Geometry: final body of the model. Coordinates: model frame, mm. Face numbers are marked on the shaded views. A direction names the side the tool comes from. Give positions to 0.01 mm unless a question says otherwise; leave off trailing zeros. Write each loop counter-clockwise with the first axis right and the second up, starting at its lowest first coordinate (ties: lowest second). Pieces come first, ordered by that corner, then holes. Notation, with made-up numbers: M -4.75,-31 L 5.25,-31 A21 ccw 5.25,8 Z; hole C 42,56 d11. An arc over 180 degrees is marked long. Use a Markdown table: item, result. Add a question column.
(1) Material intervals for L1, parallel to X at y = 13.25, z = -20; L2, parallel to X at y = 6.5, z = -23; L3, parallel to Y at x = -16, z = -36.5, sorted ascending.
(2) Cut plane A-A (z = -52). Output: boundary loops of the cut face in (x, y), plus the area to 3 significant figures.
(3) Reachability of the marked faces 1, 2, 3, 4 and 5 from +Z, -Z, +X, -X, +Y, -Y: full face, straight path, thin tool, end or side. Return the list, or none.
(4) Cut plane D-D (z = -36). Output: boundary loops of the cut face in (x, y), plus the area to 3 significant figures.
(5) Cut plane C-C (y = 93). Output: boundary loops of the cut face in (x, z), plus the area to 3 significant figures.
(6) Cut plane B-B (x = -72). Output: boundary loops of the cut face in (y, z), plus the area to 3 significant figures.
(7) Pin query (flat end, axial travel): pin 1 Ø5 at (y, z) = (49.5, -51.5) entering from +X; pin 2 Ø19 at (y, z) = (46, -19.5) entering from +X; pin 3 Ø5 at (y, z) = (37.5, -32.5) entering from -X. Return the tip coordinate at first contact, or that it passes through.
(8) Draft query along X for the marked faces 6, 7, 8 and 9. Return one class per face: released by +X, released by -X, zero draft, split by the parting line, or undercut.
```python
from build123d import *

# Parameters (mm, degrees)
SKETCH2_R           = 10
BOSS_EXTRUDE1_DEPTH = 20
SKETCH3_W           = 120
SKETCH3_H           = 8
CUT_EXTRUDE1_DEPTH  = 4
SKETCH7_R           = 10
BOSS_EXTRUDE2_DEPTH = 16
BOSS_EXTRUDE3_START = 8
SKETCH8_R           = 24
SKETCH8_R_2         = 10
BOSS_EXTRUDE3_DEPTH = 8
RIB4_REACH          = 153.895
SKETCH9_WALL_W      = 381.261249794
SKETCH9_WALL_H      = 12
FILLET2_R           = 1


with BuildPart() as part:
    # Sketch2 → Boss-Extrude1 (new body)
    with BuildSketch(Plane(origin=(0, 0, 0), x_dir=(1, 0, 0), z_dir=(0, 1, 0))):
        with BuildLine():
            Line((-64.708154955, 0), (15.291845045, 0))
            ThreePointArc((15.291845045, 0), (29.433980669, 5.857864376), (35.291845045, 20))
            Line((35.291845045, 20), (35.291845045, 64))
            Line((35.291845045, 64), (-84.708154955, 64))
            Line((-84.708154955, 64), (-84.708154955, 20))
            ThreePointArc((-84.708154955, 20), (-78.850290578, 5.857864376), (-64.708154955, 0))
        make_face()
        with Locations(Location((-64.708154955, 20, 0), (0, 0, 270))):
            Circle(SKETCH2_R, mode=Mode.SUBTRACT)
        with Locations(Location((15.291845045, 20, 0), (0, 0, 270))):
            Circle(SKETCH2_R, mode=Mode.SUBTRACT)
    extrude(amount=BOSS_EXTRUDE1_DEPTH)

    # Sketch3 → Cut-Extrude1 (cut)
    with BuildSketch(Plane(origin=(0, 20, 0), x_dir=(1, 0, 0), z_dir=(0, 1, 0))):
        with Locations((-24.708154955, 60)):
            Rectangle(SKETCH3_W, SKETCH3_H)
    extrude(amount=-CUT_EXTRUDE1_DEPTH, mode=Mode.SUBTRACT)

    # Sketch7 → Boss-Extrude2 (add)
    with BuildSketch(Plane(origin=(0, 0, -56), x_dir=(-1, 0, 0), z_dir=(0, 0, -1))):
        with BuildLine():
            Line((24.708154955, 20), (54.708154955, 20))
            ThreePointArc((54.708154955, 20), (50.465514267, 21.757359313), (48.708154955, 26))
            Line((48.708154955, 26), (48.708154955, 100))
            ThreePointArc((48.708154955, 100), (24.708154955, 124), (0.708154955, 100))
            Line((0.708154955, 100), (0.708154955, 26))
            ThreePointArc((0.708154955, 26), (-1.049204358, 21.757359313), (-5.291845045, 20))
            Line((-5.291845045, 20), (24.708154955, 20))
        make_face()
        with Locations((24.708154955, 100)):
            Circle(SKETCH7_R, mode=Mode.SUBTRACT)
    extrude(amount=-BOSS_EXTRUDE2_DEPTH)

    # Sketch8 → Boss-Extrude3 (add)
    with BuildSketch(Plane(origin=(0, 0, -56), x_dir=(-1, 0, 0), z_dir=(0, 0, -1)).offset(BOSS_EXTRUDE3_START)):
        with Locations((24.708154955, 100)):
            Circle(SKETCH8_R)
        with Locations((24.708154955, 100)):
            Circle(SKETCH8_R_2, mode=Mode.SUBTRACT)
    extrude(amount=-BOSS_EXTRUDE3_DEPTH)

    # Sketch9 wall → Rib4 (add, up to next)
    with BuildSketch(Plane(origin=(-24.708154955, 52, -20), x_dir=(0, 0.847998304005, -0.529998940003), z_dir=(0, -0.529998940003, -0.847998304005)), mode=Mode.PRIVATE) as rib4_sk1:
        Rectangle(SKETCH9_WALL_W, SKETCH9_WALL_H)
    rib4_tool1 = extrude(rib4_sk1.sketch, amount=RIB4_REACH, mode=Mode.PRIVATE) - part.part
    add(rib4_tool1.solids().sort_by_distance((-24.708154955, 52, -20))[0])

    # Fillet2
    fillet2_edges = [part.edges().sort_by_distance(p)[0] for p in [
        (-6.708154955, 20, -40),
        (-42.708154955, 20, -40),
        (-24.708154955, 84, -40),
        (-30.708154955, 20, -20),
        (-30.708154955, 52, -40),
        (-18.708154955, 52, -40),
        (-18.708154955, 20, -20),
    ]]
    fillet(fillet2_edges, radius=FILLET2_R)


solid = part.part
```
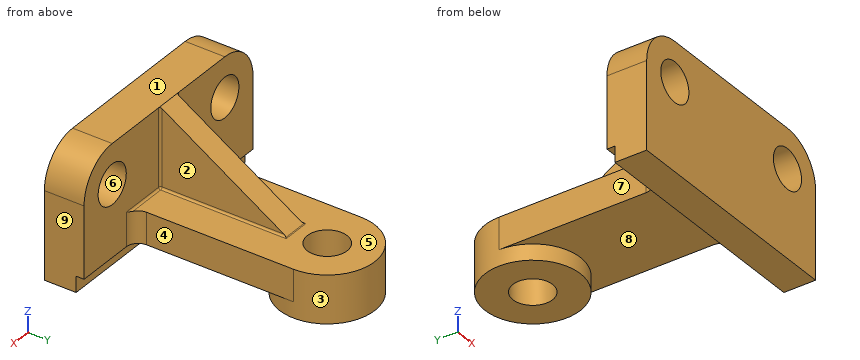
Answer list:
| question | item | result |
|---|---|---|
| 1 | L1 | -84.71 to -74.71, -54.71 to 5.29, 25.29 to 35.29 |
| 1 | L2 | -84.71 to -74.25, -55.17 to 5.75, 24.83 to 35.29 |
| 1 | L3 | 0 to 20 |
| 2 | outline | M -84.71,0 L 35.29,0 L 35.29,20 L 5.29,20 A6 cw -0.71,26 L -0.71,100 A24 ccw -48.71,100 L -48.71,26 A6 cw -54.71,20 L -84.71,20 Z; hole C -24.71,100 d20 |
| 2 | area | 6,850 mm² |
| 3 | face 1 | +Z, +X, -X, +Y, -Y |
| 3 | face 2 | +Z, +X, +Y |
| 3 | face 3 | -Z |
| 3 | face 4 | +Z, -Z, +X, +Y |
| 3 | face 5 | +Z, +Y |
| 4 | outline | M -84.71,0 L 35.29,0 L 35.29,20 L -17.71,20 A1 cw -18.71,21 L -18.71,77.6 L -30.71,77.6 L -30.71,21 A1 cw -31.71,20 L -84.71,20 Z |
| 4 | area | 3,090 mm² |
| 5 | outline | M -48.71,-56 L -47.66,-56 L -47.66,-64 L -31.85,-64 L -31.85,-40 L -48.71,-40 Z; M -17.57,-64 L -1.75,-64 L -1.75,-56 L -0.71,-56 L -0.71,-40 L -17.57,-40 Z |
| 5 | area | 793 mm² |
| 6 | outline | M 0,-64 L 16,-64 L 16,-56 L 20,-56 L 20,-26.84 L 0,-26.84 Z; M 0,-13.16 L 20,-13.16 L 20,-1.38 L 0,-1.38 Z |
| 6 | area | 947 mm² |
| 7 | pin 1 | x = -0.71 |
| 7 | pin 2 | x = -18.71 |
| 7 | pin 3 | x = -30.71 |
| 8 | face 6 | undercut |
| 8 | face 7 | released by -X |
| 8 | face 8 | zero draft |
| 8 | face 9 | released by +X |
